Could you check a few things on this drawing? It's one solid part, dimensions in mm from its lowest x, y, z. Give positions to 0.01 mm unless a question says otherwise; leave off trailing zeros. Order: outer loops, then holes, each group sorted by start corner. A loop starts at its lowest first (then second) coordinate and runs counter-clockwise, first axis right, second up. Notation, with made-up numbers: (71.5, -36.75) -> (124.5, -36.75) arc R34 cw to (124.5, -3.75) -> close; hole circle Ø1 at (-22.75, 39). An arc over 180 degrees is marked (long way). Write each question's results on one line, items separated by ' | '. Start each with the question number.
Q1. Imagine slicing it at C-C, the plane z = 46.5. Please give me the cut outline in (x, y), then the cut area to 3 significant figures.
Q2. Imagine slicing it at A-A, the plane y = 0.8. State how many separate pieces and enclosed holes the cut face has, then the cut area to 3 significant figures.
Q3. I'm going to push flat-ended pins straight in: pin 1 (0.6 mm diameter, centred on x = 3.5, y = 1, fed in from -Z); pin 2 (1 mm diameter, centred on x = 85, y = 1.5, fed in from +Z); pin 3 (1 mm diameter, centred on y = 1.5, z = 86, fed in from +X). Where does each tip first touch, or does it pass through?
Q4. Imagine slicing it at D-D, the plane x = 14.5. Please give me the cut outline in (y, z).
Q5. I need wall thicknesses on line 1 along Z through (x, y) = (58.5, 1.05) (1 decimal); line 2 along Z through (x, y) = (82.5, 1.2) (1 decimal); line 3 along X through (y, z) = (0.25, 5). Which ranges of each line are inside material? Lowest first, please. Write a range as [from, to].
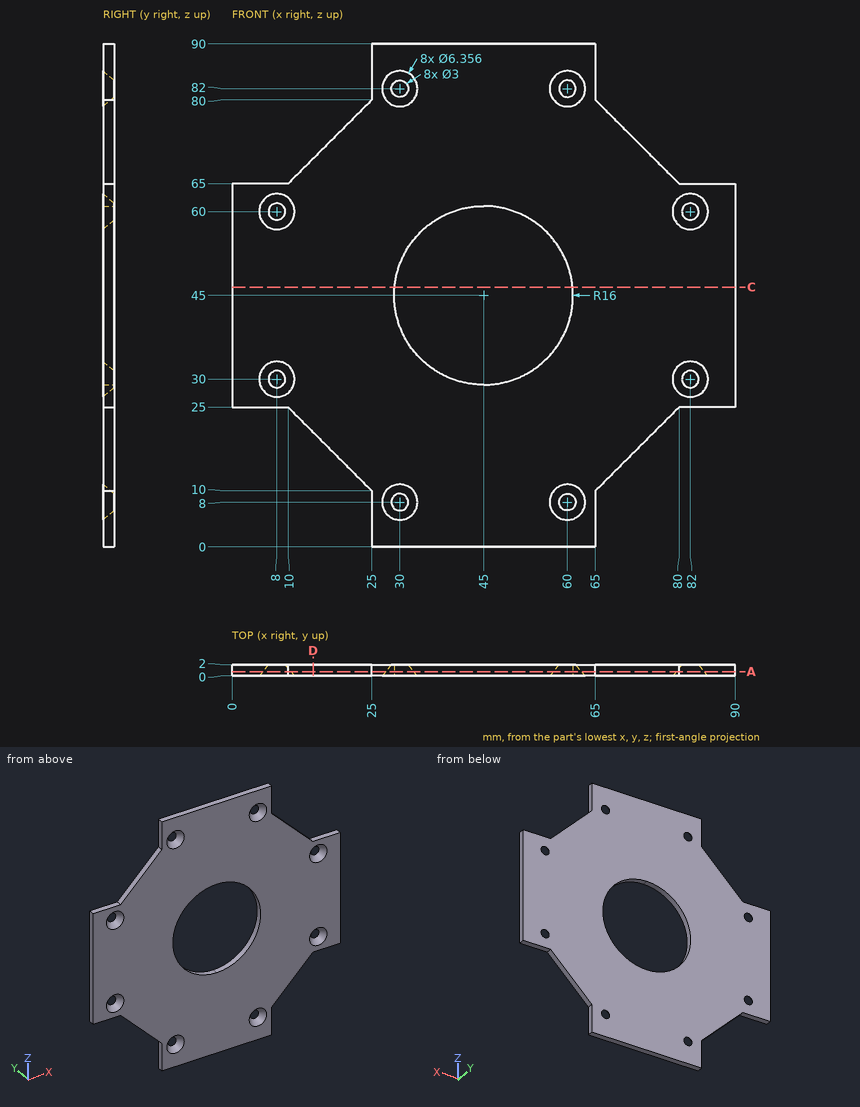
Geometry check:
1) outline: (0, 0) -> (29.07, 0) -> (29.07, 2) -> (0, 2) -> close; (60.93, 0) -> (90, 0) -> (90, 2) -> (60.93, 2) -> close | area: 116 mm²
2) separate pieces: 1 | enclosed holes: 9 | area: 5,090 mm²
3) pin 1: z = 25 | pin 2: z = 65 | pin 3: x = 65
4) outline: (0, 20.5) -> (2, 20.5) -> (2, 69.5) -> (0, 69.5) -> close
5) line 1: [0, 6.3], [9.7, 36.4], [53.6, 80.3], [83.7, 90] | line 2: [25, 27.9], [32.1, 57.9], [62.1, 65] | line 3: [25, 65]
